Read the model definition and answer for the solid it produces. Units are mm, in the model's axes. Give positions to 0.01 mm unless a question says otherwise; leave off trailing zeros. Loops run counter-clockwise (first coordinate to the right, second up) from the corner with the lowest first, then second, coordinate; pieces in that order, holes last. Notation, with made-up numbers: (28.25, -17) - (41.25, -17) arc R31 ccw to (41.25, 20) - close; hole circle Ø11 at (-39.75, 16). An arc over 180 degrees is marked (long way). Put each result on its own line as item: value. Start each with the question number.
1. A cutting plane is placed at D-D, the plane y = 42. Determine the outline of the cut face in (x, z), plus the area to 3 significant figures.
2. A cutting plane is placed at C-C, the plane x = 6.35. Count the separate pieces of the cut face and the enclosed holes in it, plus the area to 3 significant figures.
3. Given pin 1 Ø1.4 at (x, z) = (6.5, 9.5) entering from +Y; pin 2 Ø4 at (x, y) = (11, 91) entering from +Z; pin 3 Ø3 at (x, z) = (8.5, 6) entering from -Y, each flat-ended and moving along its own axis, determine where each tip first touches the part or whether it passes through.
4. A cutting plane is placed at B-B, the plane y = 22.86. Determine the outline of the cut face in (x, z), plus the area to 3 significant figures.
5. A cutting plane is placed at A-A, the plane y = 2.54. Determine the outline of the cut face in (x, z).
6. Consider L1, parallel to X at y = 22.86, z = 6; L2, parallel to Y at x = 6.35, z = -1.75; L3, parallel to Y at x = 5.08, z = -2.75 (3 decimals). Determine where each line is inside the solid, lowest interval first. Write a range as from..to.
```python
from build123d import *

# Parameters (mm, degrees)
SKETCH1_W                       = 12.7
SKETCH1_H                       = 114.3
BOSS_EXTRUDE1_DEPTH             = 6.35
SKETCH4_W                       = 12.7
SKETCH4_H                       = 28.575
BOSS_EXTRUDE3_DEPTH             = 6.35
SKETCH5_W                       = 12.7
SKETCH5_H                       = 28.575
BOSS_EXTRUDE4_DEPTH             = 6.35
SKETCH7_W                       = 6.35
SKETCH7_H                       = 19.05
CUT_EXTRUDE2_DEPTH              = 32.512
CUT_EXTRUDE3_DEPTH              = 116.702506455
CUT_EXTRUDE3_DEPTH_BACK         = 116.702506455
SKETCH8_R                       = 2.38125
FILLET5_RADIUS                  = 6.35
FILLET5_LENGTH                  = 6.35
SKETCH9_W                       = 12.7
SKETCH9_H                       = 6.35
BOSS_EXTRUDE5_DEPTH             = 6.35
FILLET6_R                       = 2.54
F_3_16_0_1875_DOWEL_HOLE1_D     = 4.7625
F_3_16_0_1875_DOWEL_HOLE1_DEPTH = 23.368
F_3_16_0_1875_DOWEL_HOLE1_TIP   = 1.430799349


with BuildPart() as part:
    # Sketch1 → Boss-Extrude1 (new body)
    with BuildSketch(Plane.XY):
        with Locations((6.35, 57.15)):
            Rectangle(SKETCH1_W, SKETCH1_H)
    extrude(amount=BOSS_EXTRUDE1_DEPTH)

    # Sketch4 → Boss-Extrude3 (add)
    with BuildSketch(Plane.XY.offset(6.35)):
        with Locations((6.35, 14.2875)):
            Rectangle(SKETCH4_W, SKETCH4_H)
    extrude(amount=BOSS_EXTRUDE3_DEPTH)

    # Sketch5 → Boss-Extrude4 (add)
    with BuildSketch(Plane(origin=(0, 0, 0), x_dir=(-1, 0, 0), z_dir=(0, 0, -1))):
        with Locations((-6.35, 14.2875)):
            Rectangle(SKETCH5_W, SKETCH5_H)
    extrude(amount=BOSS_EXTRUDE4_DEPTH)

    # Sketch7 → Cut-Extrude2 (cut)
    with BuildSketch(Plane.ZY):
        with Locations((3.175, 9.525)):
            Rectangle(SKETCH7_W, SKETCH7_H)
    extrude(amount=-CUT_EXTRUDE2_DEPTH, mode=Mode.SUBTRACT)

    # Sketch8 → Cut-Extrude3 (cut, two sides: drawn at the far end of the back side and taken through both)
    with BuildSketch(Plane.XY.offset(6.35).offset(-CUT_EXTRUDE3_DEPTH_BACK)):
        with Locations((6.35, 22.86)):
            Circle(SKETCH8_R)
    extrude(amount=CUT_EXTRUDE3_DEPTH + CUT_EXTRUDE3_DEPTH_BACK, mode=Mode.SUBTRACT)

    # Fillet5: full round fillet: the end face becomes a half cylinder, R = half its width
    fillet5_face = Plane((6.35, 114.3, 3.175), x_dir=(0, 0, 1), z_dir=(0, 1, 0))  # on the end face: x along it, z out of the body
    fillet5_slab = fillet5_face.offset(-FILLET5_RADIUS / 2) * Box(FILLET5_LENGTH, 2 * FILLET5_RADIUS, FILLET5_RADIUS, mode=Mode.PRIVATE)  # the body's end, R deep
    fillet5_round = Plane((6.35, 107.95, 3.175), x_dir=(0, 1, 0), z_dir=(0, 0, 1)) * Cylinder(FILLET5_RADIUS, FILLET5_LENGTH, mode=Mode.PRIVATE)  # its axis R under the face
    add(fillet5_slab - fillet5_round, mode=Mode.SUBTRACT)

    # Sketch9 → Boss-Extrude5 (add)
    with BuildSketch(Plane.XZ):
        with Locations((6.35, -3.175)):
            Rectangle(SKETCH9_W, SKETCH9_H)
        with Locations((6.35, 9.525)):
            Rectangle(SKETCH9_W, SKETCH9_H)
    extrude(amount=BOSS_EXTRUDE5_DEPTH)

    # Fillet6
    fillet6_edges = [part.edges().sort_by_distance(p)[0] for p in [
        (12.7, 68.2625, 6.35),
        (0, 28.575, 9.525),
        (6.35, 28.575, 6.35),
        (12.7, 28.575, 9.525),
        (0, 11.1125, 12.7),
        (12.7, 11.1125, 12.7),
        (6.35, 28.575, 12.7),
        (12.7, 68.2625, 0),
        (12.7, 28.575, -3.175),
        (6.35, 28.575, 0),
        (0, 28.575, -3.175),
        (12.7, 14.2875, -6.35),
        (0, 14.2875, -6.35),
        (6.35, 28.575, -6.35),
        (12.7, 9.525, 6.35),
        (12.7, 19.05, 3.175),
        (12.7, 9.525, 0),
        (0, 9.525, 0),
        (0, 9.525, 6.35),
        (0, 19.05, 3.175),
        (0, 68.2625, 6.35),
        (0, 68.2625, 0),
        (6.35, 114.3, 0),
        (6.35, 114.3, 6.35),
        (6.35, -6.35, -6.35),
        (12.7, -6.35, -3.175),
        (6.35, -6.35, 0),
        (0, -6.35, -3.175),
        (6.35, -6.35, 12.7),
        (0, -6.35, 9.525),
        (6.35, -6.35, 6.35),
        (12.7, -6.35, 9.525),
    ]]
    fillet(fillet6_edges, radius=FILLET6_R)

    # 3/16 (0.1875) Dowel Hole1
    with Locations(Plane.XY.offset(12.7)):
        with Locations((5.08, 2.54)):
            Hole(F_3_16_0_1875_DOWEL_HOLE1_D / 2, depth=F_3_16_0_1875_DOWEL_HOLE1_DEPTH)
            with Locations((0, 0, -(F_3_16_0_1875_DOWEL_HOLE1_DEPTH + F_3_16_0_1875_DOWEL_HOLE1_TIP / 2))):  # 118° drill point
                Cone(0, F_3_16_0_1875_DOWEL_HOLE1_D / 2, F_3_16_0_1875_DOWEL_HOLE1_TIP, mode=Mode.SUBTRACT)


solid = part.part
```
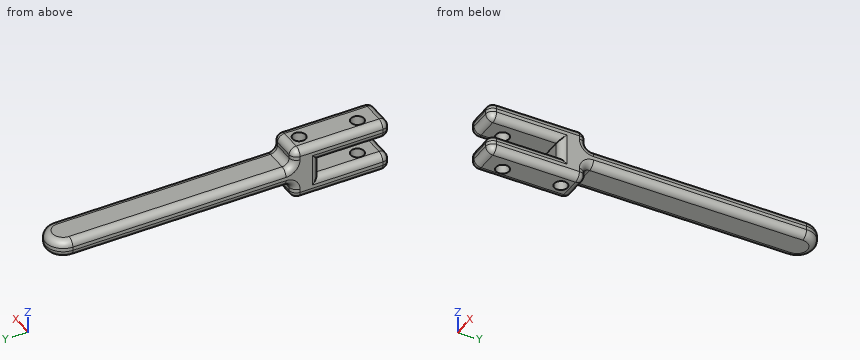
Return value:
1. outline: (0, 2.54) arc R2.54 ccw to (2.54, 0) - (10.16, 0) arc R2.54 ccw to (12.7, 2.54) - (12.7, 3.81) arc R2.54 ccw to (10.16, 6.35) - (2.54, 6.35) arc R2.54 ccw to (0, 3.81) - close
1. area: 75.1 mm2
2. separate pieces: 4
2. enclosed holes: 0
2. area: 898 mm2
3. pin 1: stops at y = 28.58
3. pin 2: stops at z = 6.35
3. pin 3: stops at y = -5.94
4. outline: (0, -3.81) arc R2.54 ccw to (2.54, -6.35) - (3.97, -6.35) - (3.97, 12.7) - (2.54, 12.7) arc R2.54 ccw to (0, 10.16) - close; (8.73, -6.35) - (10.16, -6.35) arc R2.54 ccw to (12.7, -3.81) - (12.7, 10.16) arc R2.54 ccw to (10.16, 12.7) - (8.73, 12.7) - close
4. area: 146 mm2
5. outline: (0, -3.81) arc R2.54 ccw to (2.54, -6.35) - (2.7, -6.35) - (2.7, 0) - (2.54, 0) arc R2.54 ccw to (0, -2.54) - close; (0, 8.89) arc R2.54 ccw to (2.54, 6.35) - (2.7, 6.35) - (2.7, 12.7) - (2.54, 12.7) arc R2.54 ccw to (0, 10.16) - close; (7.46, -6.35) - (10.16, -6.35) arc R2.54 ccw to (12.7, -3.81) - (12.7, -2.54) arc R2.54 ccw to (10.16, 0) - (7.46, 0) - close; (7.46, 6.35) - (10.16, 6.35) arc R2.54 ccw to (12.7, 8.89) - (12.7, 10.16) arc R2.54 ccw to (10.16, 12.7) - (7.46, 12.7) - close
6. L1: x = 0..3.97, 8.73..12.7
6. L2: y = -6.22..0.53, 4.55..20.48, 25.24..28.7
6. L3: y = -6.35..0.159, 4.921..20.846, 24.874..28.575
